CAD build for the part. Positions are in the model's coordinates, mm. Coordinates: 2 decimals unless noted, no trailing zeros. Write each loop counter-clockwise with the first axis right and the second up, starting at its lowest first coordinate (ties: lowest second). Pieces come first, ordered by that corner, then holes. Notation, with made-up numbers: (-37.75, 24) -> (-4.75, 24) arc R22 ccw to (-4.75, 56) -> close; hole circle Ø7 at (-32.75, 4.5). An arc over 180 degrees is marked (long way). Answer as CSV lines item,"result". Start each with the question number.
Autodesk Inventor part; units mm, degrees
ref_plane "YZ Plane" through (0, 0, 0) normal (1, 0, 0) x (0, 1, 0)
ref_plane "XZ Plane" through (0, 0, 0) normal (0, 1, 0) x (-1, 0, 0)
ref_plane "XY Plane" through (0, 0, 0) normal (0, 0, 1) x (1, 0, 0)
sketch "Sketch1" plane through (0, 0, 0) normal (0, 1, 0) x (-1, 0, 0)
  line L0 (0, 0) -> (101.6, 0)
  line L1 (101.6, 0) -> (101.6, -241.3)
  line L2 (101.6, -241.3) -> (0, -241.3)
  line L3 (0, -241.3) -> (0, 0)
  dimension "d0" = 101.6
  dimension "d1" = 241.3
extrude "Extrusion1" add sketch "Sketch1" along normal blind 19.05
hole "Hole1" at (-47.625, 0, -180.975) direction (0, 1, 0) diameter 50.8 end through all
hole "Hole2" at (-47.625, 0, -60.325) direction (0, 1, 0) diameter 50.8 end through all
sketch "Sketch3" plane through (-101.6, 0, 0) normal (0, 0, 1) x (1, 0, 0)
  line L0 (18.0708, 8.9693) -> (0.9487, 0.6183)
  line L1 (0.9487, 0.6183) -> (0, 0.1556)
  line L2 (0, 0) -> (0, 19.05)
  line L3 (18.0708, 8.9693) -> (38.7393, 19.05)
  line L4 (0, 19.05) -> (101.6, 19.05)
  line L5 (38.7393, 19.05) -> (0, 19.05)
  point P0 (101.6, 0)
extrude "Extrusion3" cut sketch "Sketch3" against normal blind 241.3
properties part number "top_slant"
1. Cut at D-D (z = -226). Give the cut face in (x, y).
2. Cut at B-B (z = -181). Give the cut face in (x, y).
3. Mould opens along Z. For faces 1 (the face through (-24, 19.05, -119)), 2 (the face through (-25.091, 9.658, -192.696)), 3 (the face through (-39, 9, 0)) say: pulls with the +Z half, pulls with the -Z half, needs draft (parallel to the pull), parting line crosses it, or undercut.
4. Cut at A-A (x = -36.5). Give the cut face in (y, z), then the cut area to 3 significant figures.
5. Flat gauge pins, fed straight in: P1, Ø1, axis at y = 9.5, z = -79, coming from the -X side; P2, Ø3, axis at y = 5, z = -104.5, coming from the -X side; P3, Ø5, axis at y = 13, z = -175.5, coming from the -X side; P4, Ø6, axis at x = -48.5, z = -80, coming from the +Y side. Where does each tip first touch, or does it go through?
6. Wall check: line 1 (Z direction, x = -46.5, y = 14.75); line 2 (Z direction, x = -68, y = 1.5); line 3 (X direction, y = 12.5, z = -163.5). Give the ranges that are in metal, low to high.
7. Cut at C-C (y = 4). Give the cut face in (x, z) (3 decimals).
Geometry check:
1,outline,"(-101.6, 0) -> (0, 0) -> (0, 19.05) -> (-62.86, 19.05) -> (-83.53, 8.97) -> (-100.65, 0.62) -> (-101.6, 0.16) -> close"
2,outline,"(-101.6, 0) -> (-73.02, 0) -> (-73.02, 14.09) -> (-83.53, 8.97) -> (-100.65, 0.62) -> (-101.6, 0.16) -> close; (-22.23, 0) -> (0, 0) -> (0, 19.05) -> (-22.23, 19.05) -> close"
3,face 1,"needs draft"
3,face 2,"undercut"
3,face 3,"pulls with the +Z half"
4,outline,"(0, -241.3) -> (19.05, -241.3) -> (19.05, -203.81) -> (0, -203.81) -> close; (0, -158.14) -> (19.05, -158.14) -> (19.05, -83.16) -> (0, -83.16) -> close; (0, -37.49) -> (19.05, -37.49) -> (19.05, 0) -> (0, 0) -> close"
4,area,"2,860 mm²"
5,P1,"x = -83.47"
5,P2,"x = -94.74"
5,P3,"x = -80.39"
5,P4,"through"
6,line 1,"-241.3 to -206.35, -155.6 to -85.7, -34.95 to 0"
6,line 2,"-241.3 to -196.14, -165.81 to -75.49, -45.16 to 0"
6,line 3,"-76.29 to -66.06, -29.19 to 0"
7,outline,"(-93.718, -241.3) -> (0, -241.3) -> (0, 0) -> (-93.718, 0) -> close; hole circle Ø50.8 at (-47.625, -180.975); hole circle Ø50.8 at (-47.625, -60.325)"
